```python
from build123d import *

# Parameters (mm, degrees)
F2_R     = 1.5875
F3_DEPTH = 130.176
F4_R     = 3.175
F5_DEPTH = 25.4


with BuildPart() as f1:
    # F0 (on Front) → F1 (revolve)
    with BuildSketch(Plane.XZ):
        Polygon((0, -53.975), (0, 0), (0, 76.2), (-6.35, 76.2), (-6.35, 0), (-12.7, 0), align=None)
    revolve(axis=Axis((0, 0, 38.1), (0, 0, -1)))

    # F2 (on face) → F3 (cut, through all)
    with BuildSketch(Plane.XY.offset(76.2)):
        Circle(F2_R)
    extrude(amount=-F3_DEPTH, mode=Mode.SUBTRACT)

    # F4 (on face) → F5 (cut)
    with BuildSketch(Plane.XY.offset(76.2)):
        Circle(F4_R)
    extrude(amount=-F5_DEPTH, mode=Mode.SUBTRACT)


solid = f1.part
```
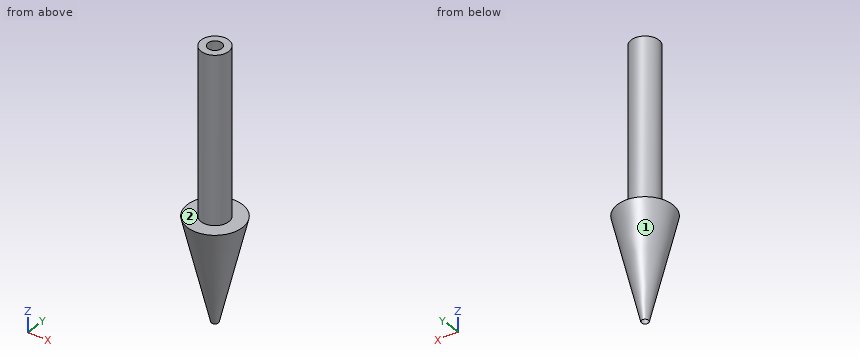
For this review, take the finished solid that the model builds, in its own axes (mm). Face numbers are marked on the shaded views. A direction names the side the tool comes from. Round coordinates to 2 decimals unless told otherwise and drop trailing zeros. Write each loop counter-clockwise with the first axis right and the second up, starting at its lowest first coordinate (ties: lowest second). Pieces come first, ordered by that corner, then holes. Notation, with made-up numbers: (10.5, 31.25) - (60.5, 31.25) arc R31 cw to (60.5, 68.25) - close; hole circle Ø10 at (48.5, 55.25). An arc over 180 degrees is marked (long way). Answer as a JSON object with one key per item and string values.
1. We need section C-C on z = 59. Give the boundary of the cut face in (x, y) (3 decimals).
Response values:
{"outline": "circle Ø12.7 at (0, 0); hole circle Ø6.35 at (0, 0)"}
2. To check wall thickness, follow line 1 along Y through (x, z) = (0, 57) (3 decimals); line 2 along Y through (x, z) = (0, 7); line 3 along X through (y, z) = (0, -12.5). State the ranges of each line that lie inside material, in increasing order.
Response values:
{"line 1": "y = -6.35 to -3.175, 3.175 to 6.35", "line 2": "y = -6.35 to -1.59, 1.59 to 6.35", "line 3": "x = -9.76 to -1.59, 1.59 to 9.76"}
3. Tool access review of the marked faces 1 and 2: name each direction out of +Z, -Z, +X, -X, +Y, -Y from which nothing blocks a thin tool from reaching the whole face with its end or side.
Response values:
{"face 1": "-Z", "face 2": "+Z"}
4. For pin 1 Ø3 at (x, y) = (3.5, -9) entering from +Z; pin 2 Ø6 at (y, z) = (4.5, -10.5) entering from +X; pin 3 Ø10 at (x, z) = (-5, -14) entering from -Y; pin 4 Ø4 at (y, z) = (-9, 58) entering from -X, all flat-tipped, find the tip position at first contact; note any pin that passes through.
Response values:
{"pin 1": "stops at z = 0", "pin 2": "stops at x = 10.46", "pin 3": "stops at y = -10.15", "pin 4": "passes through"}
